For this review, take the finished solid that the model builds, in its own axes (mm). Coordinates: 2 decimals unless noted, no trailing zeros. Write each loop counter-clockwise with the first axis right and the second up, starting at its lowest first coordinate (ties: lowest second). Pieces come first, ordered by that corner, then holes. Notation, with made-up numbers: (5, 53) -> (41, 53) arc R24 ccw to (41, 91) -> close; hole circle Ø7 at (26, 1). An arc over 180 degrees is marked (long way). Put each result on its own line as item: value. Start each with the question number.
Item 1: Consider section B-B on y = 12.7. Give the boundary of the cut face in (x, z), and give its area (3 significant figures).
Item 2: Consider section C-C on z = 43. Give the boundary of the cut face in (x, y).
Item 3: Consider section D-D on y = -5. Give the boundary of the cut face in (x, z).
Item 4: The part is to be moulded in two halves that separate along X. For faces 1 (the cylindrical face through (-11.722, -15.058, 1.503)), 2 (the flat face through (-28.448, 0, 31)), 3 (the cylindrical face through (-29.99, -10.21, 19.35)), say which applies: +X half, -X half, draft (parallel to the pull), parting line (faces both ways), or undercut.
Item 5: To check wall thickness, follow L1, parallel to Y at x = 12.7, z = 2.15; L2, parallel to X at y = 12, z = 1; L3, parallel to X at y = -12.7, z = 2.2. State the ranges of each line that lie inside material, in increasing order.
Item 6: Insertion check: P1, Ø1, axis at y = -14.5, z = 6, coming from the +X side; P2, Ø8, axis at x = -7.5, y = -4.5, coming from the +Z side; P3, Ø4.5, axis at x = -12.7, y = 12.7, coming from the +Z side. Each pin has a flat end and moves straight along its axis. Give the tip position at first contact, or say it passes through.
Item 7: Consider section A-A on x = 12.7. Give the boundary of the cut face in (y, z), and give its area (3 significant figures).
Autodesk Inventor part; units mm, degrees
ref_plane "YZ Plane" through (0, 0, 0) normal (1, 0, 0) x (0, 1, 0)
ref_plane "XZ Plane" through (0, 0, 0) normal (0, 1, 0) x (-1, 0, 0)
ref_plane "XY Plane" through (0, 0, 0) normal (0, 0, 1) x (1, 0, 0)
sketch "Sketch1" plane through (0, 0, 0) normal (0, 0, 1) x (1, 0, 0)
  line L0 (25.4, 25.4) -> (-25.4, 25.4)
  line L1 (-25.4, 25.4) -> (-25.4, -25.4)
  line L2 (-25.4, -25.4) -> (25.4, -25.4)
  line L3 (25.4, -25.4) -> (25.4, 25.4)
  line L4 (25.4, 25.4) -> (-25.4, -25.4) construction
  line L5 (-25.4, 25.4) -> (25.4, -25.4) construction
  point P0 (0, 0)
  dimension "d0" = 50.8
  dimension "d1" = 50.8
extrude "Plate1" add sketch "Sketch1" along normal blind 3.048
sketch "Sketch2" plane through (-28.448, -25.4, 6.096) normal (-1, 0, 0) x (0, -1, 0)
  line L0 (-50.8, 0) -> (0, 0)
  line L1 (0, 0) -> (0, 50.8)
  line L2 (0, 50.8) -> (-50.8, 50.8)
  line L3 (-50.8, 50.8) -> (-50.8, 0)
edge flange "Flange1" height 56.896 angle 90 thickness 3.048 bend radius 3.048 thickness toward (-1, 0, 0) relief tear relief width 3.048 relief depth 1.524 edges at (-25.4, 0, 3.048) wall of the first edge with corners at (-28.448, 25.4, 6.096) (-28.448, -25.4, 6.096) (-28.448, -25.4, 56.896) (-28.448, 25.4, 56.896)
bend "Bend1"
corner "Corner1"
sketch "Sketch3" plane through (-28.448, -25.4, 56.896) normal (1, 0, 0) x (0, 0, -1)
  line L0 (50.8, 0) -> (50.8, 50.8) construction
  line L1 (0, 50.8) -> (50.8, 50.8) construction
  line L2 (0, 50.8) -> (0, 0) construction
  line L3 (0, 0) -> (50.8, 0) construction
  point P0 (56.896, 25.4)
  point P1 (38.1, 38.1)
  point P2 (38.1, 12.7)
  point P3 (12.7, 38.1)
  point P4 (12.7, 12.7)
  dimension "d13" = 12.7
  dimension "d14" = 12.7
  dimension "d17" = 25.4
  dimension "d20" = 25.4
hole "Hole1" at (-28.448, 12.7, 18.796) at (-28.448, -12.7, 18.796) at (-28.448, 12.7, 44.196) at (-28.448, -12.7, 44.196) direction (-1, 0, 0) diameter 5.1054 end through all
sketch "Sketch4" plane through (0, 0, 3.048) normal (0, 0, 1) x (1, 0, 0)
  line L0 (-25.4, 25.4) -> (25.4, 25.4) construction
  line L1 (-25.4, -25.4) -> (-25.4, 25.4) construction
  line L2 (25.4, -25.4) -> (-25.4, -25.4) construction
  line L3 (25.4, 25.4) -> (25.4, -25.4) construction
  point P0 (0, 0)
  point P1 (-12.7, 12.7)
  point P2 (12.7, 12.7)
  point P3 (-12.7, -12.7)
  point P4 (12.7, -12.7)
  dimension "d30" = 12.7
  dimension "d31" = 12.7
  dimension "d34" = 25.4
  dimension "d37" = 25.4
hole "Hole2" at (-12.7, 12.7, 3.048) at (12.7, 12.7, 3.048) at (-12.7, -12.7, 3.048) at (12.7, -12.7, 3.048) direction (0, 0, -1) diameter 5.1054 end through all
fillet "Corner Round1" radius 6.35 4 edges at (-29.972, -25.4, 56.896) (-29.972, 25.4, 56.896) (25.4, 25.4, 1.524) (25.4, -25.4, 1.524)
equation "\"d28\" = Thickness"
equation "\"d2\" = Thickness"
equation "\"d3\" = BendReliefWidth"
equation "\"d4\" = BendReliefDepth"
equation "\"d5\" = MinimumRemnant"
equation "\"d6\" = TransitionRadius"
equation "\"d9\" = BendRadius"
equation "\"d10\" = CornerReliefSize"
equation "\"d11\" = GapSize"
equation "\"d12\" = JacobiRadiusSize"
equation "\"BendRadius\" = Thickness"
equation "\"BendReliefWidth\" = Thickness"
equation "\"BendReliefDepth\" = 0.5 * Thickness"
equation "\"CornerReliefSize\" = 4 * Thickness"
equation "\"MinimumRemnant\" = 2 * Thickness"
equation "\"TransitionRadius\" = BendRadius"
equation "\"JacobiRadiusSize\" = BendRadius"
equation "\"GapSize\" = Thickness"
properties part number "hopper_side_bracket" material "Aluminum 6061"
Return value:
1. outline: (-31.5, 6.1) arc R6.1 ccw to (-25.4, 0) -> (-15.25, 0) -> (-15.25, 3.05) -> (-25.4, 3.05) arc R3.05 cw to (-28.45, 6.1) -> (-28.45, 16.24) -> (-31.5, 16.24) -> close; (-31.5, 21.35) -> (-28.45, 21.35) -> (-28.45, 41.64) -> (-31.5, 41.64) -> close; (-31.5, 46.75) -> (-28.45, 46.75) -> (-28.45, 56.9) -> (-31.5, 56.9) -> close; (-10.15, 0) -> (10.15, 0) -> (10.15, 3.05) -> (-10.15, 3.05) -> close; (15.25, 0) -> (25.4, 0) -> (25.4, 3.05) -> (15.25, 3.05) -> close
1. area: 269 mm^2
2. outline: (-31.5, -25.4) -> (-28.45, -25.4) -> (-28.45, -14.96) -> (-31.5, -14.96) -> close; (-31.5, -10.44) -> (-28.45, -10.44) -> (-28.45, 10.44) -> (-31.5, 10.44) -> close; (-31.5, 14.96) -> (-28.45, 14.96) -> (-28.45, 25.4) -> (-31.5, 25.4) -> close
3. outline: (-31.5, 6.1) arc R6.1 ccw to (-25.4, 0) -> (25.4, 0) -> (25.4, 3.05) -> (-25.4, 3.05) arc R3.05 cw to (-28.45, 6.1) -> (-28.45, 56.9) -> (-31.5, 56.9) -> close
4. face 1: undercut
4. face 2: +X half
4. face 3: draft
5. L1: -25.4 to -15.25, -10.15 to 10.15, 15.25 to 25.4
5. L2: -28.75 to -15.15, -10.25 to 10.25, 15.15 to 25.4
5. L3: -30.09 to -15.25, -10.15 to 10.15, 15.25 to 25.4
6. P1: x = -28.39
6. P2: z = 3.05
6. P3: through
7. outline: (-25.4, 0) -> (-15.25, 0) -> (-15.25, 3.05) -> (-25.4, 3.05) -> close; (-10.15, 0) -> (10.15, 0) -> (10.15, 3.05) -> (-10.15, 3.05) -> close; (15.25, 0) -> (25.4, 0) -> (25.4, 3.05) -> (15.25, 3.05) -> close
7. area: 124 mm^2
